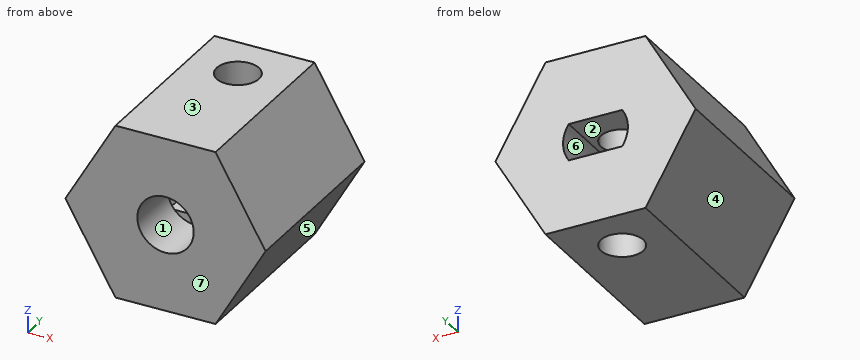
Autodesk Inventor part; units mm, degrees
ref_plane "YZ Plane" through (0, 0, 0) normal (1, 0, 0) x (0, 1, 0)
ref_plane "XZ Plane" through (0, 0, 0) normal (0, 1, 0) x (-1, 0, 0)
ref_plane "XY Plane" through (0, 0, 0) normal (0, 0, 1) x (1, 0, 0)
sketch "Sketch1" plane through (0, 0, 0) normal (0, 1, 0) x (-1, 0, 0)
  line L0 (7.1014, 0) -> (3.5507, -6.15)
  line L1 (3.5507, -6.15) -> (-3.5507, -6.15)
  line L2 (-3.5507, -6.15) -> (-7.1014, 0)
  line L3 (-7.1014, 0) -> (-3.5507, 6.15)
  line L4 (-3.5507, 6.15) -> (3.5507, 6.15)
  line L5 (3.5507, 6.15) -> (7.1014, 0)
  line L6 (0, 0) -> (25.8005, 0) construction
  dimension "d0" = 12.3
extrude "Extrusion1" add sketch "Sketch1" along normal blind 13
sketch "Sketch2" plane through (0, 13, 0) normal (0, 1, 0) x (1, 0, 0)
  line L0 (3.5507, 6.15) -> (-3.5507, 6.15)
  line L1 (-1.8974, 1.3) -> (1.8974, 1.3)
  line L2 (-1.8974, -1.3) -> (1.8974, -1.3)
  arc A0 (-1.8974, 1.3) -> (-1.8974, -1.3) centre (0, 0) ccw
  arc A1 (1.8974, -1.3) -> (1.8974, 1.3) centre (0, 0) ccw
  dimension "d4" = 2.6
  dimension "d5" = 2.3
  dimension "d6" = 2.3
extrude "Extrusion2" cut sketch "Sketch2" against normal blind 9
sketch "Sketch6" plane through (0, 0, 0) normal (0, -1, 0) x (1, 0, 0)
  circle A0 centre (0, 0) radius 2
  dimension "d16" = 4
extrude "Extrusion5" cut sketch "Sketch6" against normal up to surface (4 mm away)
sketch "Sketch7" plane through (3.5507, 0, -6.15) normal (0, 0, -1) x (-1, 0, 0)
  line L0 (0, 13) -> (7.1014, 13)
  line L1 (0, 0) -> (0, 13)
  circle A0 centre (3.5507, 9.5) radius 1.5
  line L2 (3.5507, 0) -> (3.5507, 15.2107) construction
  dimension "d19" = 3
  dimension "d20" = 3.5
extrude "Extrusion6" cut sketch "Sketch7" against normal through all
equation "\"Plastic_Reduction_Margin\" = 0.3"
properties part number "Hub_Hex_12mm" material "Polyethylene, Low Density"
Here's how the part is built. I have some questions about the finished solid (model axes, mm). Face numbers are marked on the shaded views. A direction names the side the tool comes from. Coordinates: 2 decimals unless noted, no trailing zeros. Order: outer loops, then holes, each group sorted by start corner. A loop starts at its lowest first (then second) coordinate and runs counter-clockwise, first axis right, second up. Notation, with made-up numbers: (-13, 30.25) - (46, 30.25) arc R24 cw to (46, 49.25) - close; hole circle Ø6 at (23, 76.5). An arc over 180 degrees is marked (long way). One line per question, with ' | ' between items. Start each with the question number.
1. If we mould it in two halves opening along X, with no side actions, what happens to the marked faces 4, 5, 6 and 7? For each: released by +X, released by -X, zero draft, split by the parting line, or undercut.
2. I'm going to push flat-ended pins straight in: pin 1 Ø0.6 at (x, z) = (0, -1.5) entering from -Y; pin 2 Ø1 at (y, z) = (9, -2) entering from -X; pin 3 Ø4 at (y, z) = (2, -2.5) entering from -X. Where does each tip first touch, or does it pass through?
3. If we section it at D-D (z = 3.25): Write out the boundary of the cut face in (x, y).
4. If we section it at C-C (z = 1.75): Write out the boundary of the cut face in (x, y), and give its area (3 significant figures).
5. If we section it at B-B (y = 5.75): Write out the boundary of the cut face in (x, z).
6. Which directions (+Z, -Z, +X, -X, +Y, -Y) give clear straight access to the entire face, cutting with the end or side of a thin tool? Please do the marked faces 1, 2 and 3.
7. If we section it at A-A (x = 0): Write out the boundary of the cut face in (y, z), and give its area (3 significant figures).
8. Please list where these lines run through material, in increasing order: line 1 along Z through (x, y) = (0.25, 7.25); line 2 along Y through (x, z) = (0, -3.45); line 3 along Z through (x, y) = (0, 1.3). Write a range as [from, to].
Model answer:
1) face 4: released by -X | face 5: released by +X | face 6: undercut | face 7: zero draft
2) pin 1: stops at y = 4 | pin 2: stops at x = -6.24 | pin 3: stops at x = -6.81
3) outline: (-5.23, 0) - (5.23, 0) - (5.23, 13) - (-5.23, 13) - close; hole circle Ø3 at (0, 9.5)
4) outline: (-6.09, 0) - (-0.97, 0) - (-0.97, 4) - (0.97, 4) - (0.97, 0) - (6.09, 0) - (6.09, 13) - (-6.09, 13) - close; hole circle Ø3 at (0, 9.5) | area: 144 mm²
5) outline: (-7.1, 0) - (-3.55, -6.15) - (3.55, -6.15) - (7.1, 0) - (3.55, 6.15) - (-3.55, 6.15) - close; hole (-1.9, -1.3) - (1.9, -1.3) arc R2.3 ccw to (1.9, 1.3) - (-1.9, 1.3) arc R2.3 ccw to start
6) face 1: -Y | face 2: +Y | face 3: +Z, +X, -X, +Y, -Y
7) outline: (0, -6.15) - (8, -6.15) - (8, -1.3) - (4, -1.3) - (4, -2) - (0, -2) - close; (0, 2) - (4, 2) - (4, 1.3) - (8, 1.3) - (8, 6.15) - (0, 6.15) - close; (11, -6.15) - (13, -6.15) - (13, -1.3) - (11, -1.3) - close; (11, 1.3) - (13, 1.3) - (13, 6.15) - (11, 6.15) - close | area: 91.4 mm²
8) line 1: z = [-6.15, -1.3], [1.3, 6.15] | line 2: y = [0, 8], [11, 13] | line 3: z = [-6.15, -2], [2, 6.15]
